Here's how the part is built. I have some questions about the finished solid (model axes, mm). Give positions to 0.01 mm unless a question says otherwise; leave off trailing zeros. Write each loop counter-clockwise with the first axis right and the second up, starting at its lowest first coordinate (ties: lowest second). Pieces come first, ordered by that corner, then holes. Notation, with made-up numbers: (53, 82) - (111, 82) arc R22 cw to (111, 92) - close; hole circle Ø4 at (57.25, -19.5). An arc over 180 degrees is marked (long way). One line per item, written item: value. Start each with the question number.
1) I'm going to push flat-ended pins straight in: P1, Ø1.6, axis at x = 13, z = 1.5, coming from the -Y side; P2, Ø1.6, axis at x = -4, z = 1, coming from the -Y side. Where does each tip first touch, or does it pass through?
2) Imagine slicing it at D-D on z = 3.6. Write out the boundary of the cut face in (x, y), plus the area to 3 significant figures.
3) Imagine slicing it at B-B on x = 0. Write out the boundary of the cut face in (y, z), plus the area to 3 significant figures.
4) Please list where these lines run through material, in increasing order: L1, parallel to X at y = -11.5, z = 1.5; L2, parallel to X at y = -26, z = 1.55; L3, parallel to X at y = 11, z = 4.4. Write a range as [from, to].
5) Imagine slicing it at C-C on y = 23.5. Write out the boundary of the cut face in (x, z).
6) Imagine slicing it at A-A on y = -22. Write out the boundary of the cut face in (x, z), plus the area to 3 significant figures.
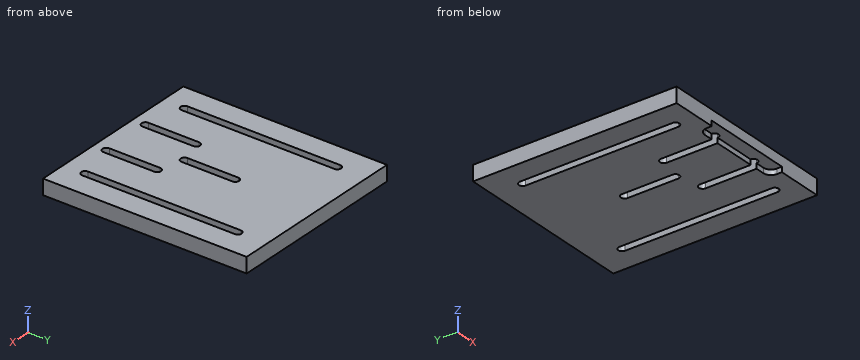
from build123d import *

# Parameters (mm, degrees)
F0_W     = 72
F0_H     = 80
F1_DEPTH = 6
F2_DEPTH = 6
F4_DEPTH = 2
F5_R     = 3


with BuildPart() as f1:
    # F0 (on Top) → F1 (new body)
    with BuildSketch(Plane.XY):
        Rectangle(F0_W, F0_H)
        with BuildLine():
            ThreePointArc((-8.5, -35), (-10, -36.5), (-11.5, -35))
            Line((-11.5, -35), (-11.5, -15))
            ThreePointArc((-11.5, -15), (-10, -13.5), (-8.5, -15))
            Line((-8.5, -15), (-8.5, -35))
        make_face(mode=Mode.SUBTRACT)
        with BuildLine():
            Line((-24, 28.5), (-24, -31.5))
            ThreePointArc((-24, -31.5), (-25.5, -33), (-27, -31.5))
            Line((-27, -31.5), (-27, 28.5))
            ThreePointArc((-27, 28.5), (-25.5, 30), (-24, 28.5))
        make_face(mode=Mode.SUBTRACT)
        with BuildLine():
            ThreePointArc((11.5, -35), (10, -36.5), (8.5, -35))
            Line((8.5, -35), (8.5, -15))
            ThreePointArc((8.5, -15), (10, -13.5), (11.5, -15))
            Line((11.5, -15), (11.5, -35))
        make_face(mode=Mode.SUBTRACT)
        with BuildLine():
            Line((-1.5, -12), (-1.5, 8))
            ThreePointArc((-1.5, 8), (0, 9.5), (1.5, 8))
            Line((1.5, 8), (1.5, -12))
            ThreePointArc((1.5, -12), (0, -13.5), (-1.5, -12))
        make_face(mode=Mode.SUBTRACT)
        with BuildLine():
            ThreePointArc((24, 28.5), (25.5, 30), (27, 28.5))
            Line((27, 28.5), (27, -31.5))
            ThreePointArc((27, -31.5), (25.5, -33), (24, -31.5))
            Line((24, -31.5), (24, 28.5))
        make_face(mode=Mode.SUBTRACT)
    extrude(amount=F1_DEPTH)

    # F0 (on Top) → F2 (cut)
    with BuildSketch(Plane.XY):
        Rectangle(F0_W, F0_H)
        with BuildLine():
            ThreePointArc((-8.5, -35), (-10, -36.5), (-11.5, -35))
            Line((-11.5, -35), (-11.5, -15))
            ThreePointArc((-11.5, -15), (-10, -13.5), (-8.5, -15))
            Line((-8.5, -15), (-8.5, -35))
        make_face(mode=Mode.SUBTRACT)
        with BuildLine():
            Line((-24, 28.5), (-24, -31.5))
            ThreePointArc((-24, -31.5), (-25.5, -33), (-27, -31.5))
            Line((-27, -31.5), (-27, 28.5))
            ThreePointArc((-27, 28.5), (-25.5, 30), (-24, 28.5))
        make_face(mode=Mode.SUBTRACT)
        with BuildLine():
            ThreePointArc((11.5, -35), (10, -36.5), (8.5, -35))
            Line((8.5, -35), (8.5, -15))
            ThreePointArc((8.5, -15), (10, -13.5), (11.5, -15))
            Line((11.5, -15), (11.5, -35))
        make_face(mode=Mode.SUBTRACT)
        with BuildLine():
            Line((-1.5, -12), (-1.5, 8))
            ThreePointArc((-1.5, 8), (0, 9.5), (1.5, 8))
            Line((1.5, 8), (1.5, -12))
            ThreePointArc((1.5, -12), (0, -13.5), (-1.5, -12))
        make_face(mode=Mode.SUBTRACT)
        with BuildLine():
            ThreePointArc((24, 28.5), (25.5, 30), (27, 28.5))
            Line((27, 28.5), (27, -31.5))
            ThreePointArc((27, -31.5), (25.5, -33), (24, -31.5))
            Line((24, -31.5), (24, 28.5))
        make_face(mode=Mode.SUBTRACT)
    extrude(amount=-F2_DEPTH, mode=Mode.SUBTRACT)

    # F3 (on face) → F4 (cut)
    with BuildSketch(Plane(origin=(0, 0, 0), x_dir=(1, 0, 0), z_dir=(0, 0, -1))):
        with BuildLine():
            Line((18, 35), (18, 40))
            Line((18, 40), (-18, 40))
            Line((-18, 40), (-18, 35))
            Line((-18, 35), (-11.5, 35))
            ThreePointArc((-11.5, 35), (-10, 36.5), (-8.5, 35))
            Line((-8.5, 35), (8.5, 35))
            ThreePointArc((8.5, 35), (10, 36.5), (11.5, 35))
            Line((11.5, 35), (18, 35))
        make_face()
    extrude(amount=-F4_DEPTH, mode=Mode.SUBTRACT)

    # F5
    f5_edges = [f1.edges().sort_by_distance(p)[0] for p in [
        (-18, -35, 1),
        (18, -35, 1),
    ]]
    fillet(f5_edges, radius=F5_R)


solid = f1.part
Numbers:
1. P1: y = -40
1. P2: y = -35
2. outline: (-36, -40) - (36, -40) - (36, 40) - (-36, 40) - close; hole (-27, -31.5) arc R1.5 ccw to (-24, -31.5) - (-24, 28.5) arc R1.5 ccw to (-27, 28.5) - close; hole (-11.5, -35) arc R1.5 ccw to (-8.5, -35) - (-8.5, -15) arc R1.5 ccw to (-11.5, -15) - close; hole (-1.5, -12) arc R1.5 ccw to (1.5, -12) - (1.5, 8) arc R1.5 ccw to (-1.5, 8) - close; hole (8.5, -35) arc R1.5 ccw to (11.5, -35) - (11.5, -15) arc R1.5 ccw to (8.5, -15) - close; hole (24, -31.5) arc R1.5 ccw to (27, -31.5) - (27, 28.5) arc R1.5 ccw to (24, 28.5) - close
2. area: 5,180 mm^2
3. outline: (-40, 2) - (-35, 2) - (-35, 0) - (-13.5, 0) - (-13.5, 6) - (-40, 6) - close; (9.5, 0) - (40, 0) - (40, 6) - (9.5, 6) - close
3. area: 332 mm^2
4. L1: [-36, -27], [-24, -1.5], [1.5, 24], [27, 36]
4. L2: [-36, -27], [-24, -11.5], [-8.5, 8.5], [11.5, 24], [27, 36]
4. L3: [-36, -27], [-24, 24], [27, 36]
5. outline: (-36, 0) - (-27, 0) - (-27, 6) - (-36, 6) - close; (-24, 0) - (24, 0) - (24, 6) - (-24, 6) - close; (27, 0) - (36, 0) - (36, 6) - (27, 6) - close
6. outline: (-36, 0) - (-27, 0) - (-27, 6) - (-36, 6) - close; (-24, 0) - (-11.5, 0) - (-11.5, 6) - (-24, 6) - close; (-8.5, 0) - (8.5, 0) - (8.5, 6) - (-8.5, 6) - close; (11.5, 0) - (24, 0) - (24, 6) - (11.5, 6) - close; (27, 0) - (36, 0) - (36, 6) - (27, 6) - close
6. area: 360 mm^2
